Model file for the job. Use its own axes, mm. Face numbers are marked on the shaded views. A direction names the side the tool comes from. Coordinates: 2 decimals unless noted, no trailing zeros. Order: outer loops, then holes, each group sorted by start corner. A loop starts at its lowest first (then second) coordinate and runs counter-clockwise, first axis right, second up. Notation, with made-up numbers: (86.25, 77.25) -> (135.25, 77.25) arc R21 ccw to (135.25, 112.25) -> close; hole circle Ø5 at (-9.5, 54). An arc over 180 degrees is marked (long way). Return JSON: item names as keys, results as strings. Group by question number.
1) Which spindle directions (+Z, -Z, +X, -X, +Y, -Y) get a long thin tool onto all of the face, cutting with end or side? Do the marked faces 1, 2 and 3. Say none if no direction does.
2) Cut at A-A (z = 10.5). Write the cut outline in (x, y), and give its area (3 significant figures).
3) Probe line 1 (Z direction, x = 27.75, y = -19.5); line 2 (Y direction, x = 18, z = 18.5); line 3 (Y direction, x = 23.25, z = 20). List the from-to ranges inside material, lowest first.
4) Cut at B-B (z = 22.5). State how many separate pieces and enclosed holes the cut face has, and give its area (3 significant figures).
5) Flat gauge pins, fed straight in: pin 1 (1.8 mm diameter, centred on x = 11.5, z = 18.5, fed in from +Y); pin 2 (4 mm diameter, centred on x = 23, z = 0.5, fed in from -Y); pin 3 (6.5 mm diameter, centred on y = -13, z = 16.5, fed in from +X). Where does each tip first touch, or does it go through?
6) Pull direction X, two halves, no side cores. Call the marked faces 4, 5, 6 and 7: +X half, -X half, draft (parallel to the pull), parting line (faces both ways), or undercut.
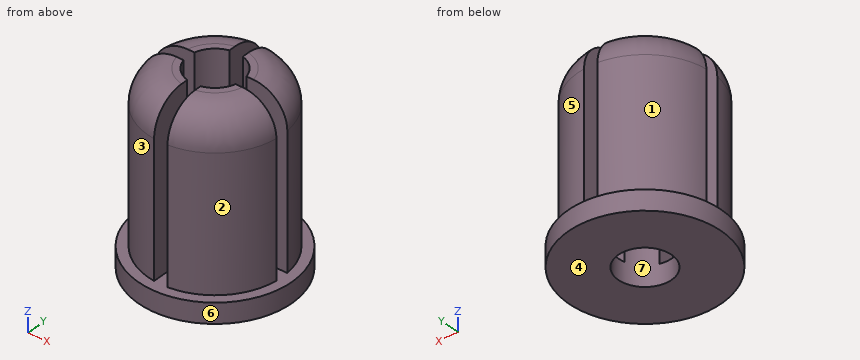
from build123d import *

# Parameters (mm, degrees)
F0_R      = 10
F0_R_2    = 4
F1_DEPTH  = 25
F2_R      = 11.5
F2_R_2    = 4
F3_DEPTH  = 3
F4_W      = 15.4053421468
F4_H      = 2
F4_W_2    = 2
F4_H_2    = 14.8476130934
F4_H_3    = 18.3621469838
F5_DEPTH  = 25
F6_R      = 5
F7_W      = 54.985769093
F7_H      = 45.2365130186
F8_DEPTH  = 25
F11_COUNT = 4
F11_ANGLE = 270


with BuildPart() as f1:
    # F0 (on Top) → F1 (new body)
    with BuildSketch(Plane.XY):
        Circle(F0_R)
        Circle(F0_R_2, mode=Mode.SUBTRACT)
    extrude(amount=F1_DEPTH)

    # F2 (on Top) → F3 (join)
    with BuildSketch(Plane.XY):
        Circle(F2_R)
        Circle(F2_R_2, mode=Mode.SUBTRACT)
    extrude(amount=-F3_DEPTH)

    # F4 (on Top) → F5 (cut)
    with BuildSketch(Plane.XY):
        with Locations((-8.7026710734, 0)):
            Rectangle(F4_W, F4_H)
        with Locations((0, 8.4238065467)):
            Rectangle(F4_W_2, F4_H_2)
        Rectangle(F4_W_2, F4_H)
        Polygon((17.6404397935, 1), (1, 1), (1, -1), (18.0223640054, -1), align=None)
        with Locations((0, -10.1810734919)):
            Rectangle(F4_W_2, F4_H_3)
    extrude(amount=F5_DEPTH, mode=Mode.SUBTRACT)

    # F6
    f6_edges = [f1.edges().sort_by_distance(p)[0] for p in [
        (7.071068, -7.071068, 25),
        (7.071068, 7.071068, 25),
        (-7.071068, 7.071068, 25),
        (-7.071068, -7.071068, 25),
    ]]
    fillet(f6_edges, radius=F6_R)


with BuildPart() as f8:
    # F7 (on Top) → F8 (new body)
    with BuildSketch(Plane.XY):
        with Locations((-82.9663015902, -56.8597912788)):
            Rectangle(F7_W, F7_H)
    extrude(amount=F8_DEPTH)


with BuildPart() as f11_1:
    # F11: instance of F1
    add(f1.part.rotate(Axis((0, -20.0353357941, 8.0697890371), (0, 0, -1)), 1 * F11_ANGLE / (F11_COUNT - 1)))


with BuildPart() as f11_2:
    # F11: instance of F1
    add(f1.part.rotate(Axis((0, -20.0353357941, 8.0697890371), (0, 0, -1)), 2 * F11_ANGLE / (F11_COUNT - 1)))


with BuildPart() as f11_3:
    # F11: instance of F1
    add(f1.part.rotate(Axis((0, -20.0353357941, 8.0697890371), (0, 0, -1)), 3 * F11_ANGLE / (F11_COUNT - 1)))


solid = f11_1.part
Answers below:
{
 "1": {"face 1": "+Z, -X, +Y", "face 2": "+Z, +X, -Y", "face 3": "+Z, -X, -Y"},
 "2": {"outline": "(10.09, -21.04) arc R10 ccw to (19.04, -29.99) -> (19.04, -23.91) arc R4 cw to (16.16, -21.04) -> close; (10.09, -19.04) -> (16.16, -19.04) arc R4 cw to (19.04, -16.16) -> (19.04, -10.09) arc R10 ccw to start; (21.04, -29.99) arc R10 ccw to (29.99, -21.04) -> (23.91, -21.04) arc R4 cw to (21.04, -23.91) -> close; (21.04, -16.16) arc R4 cw to (23.91, -19.04) -> (29.99, -19.04) arc R10 ccw to (21.04, -10.09) -> close", "area": "216 mm^2"},
 "3": {"line 1": "z = -3 to 0", "line 2": "y = -29.83 to -23.48, -16.59 to -10.24", "line 3": "y = -29.5 to -22.42, -17.66 to -10.57"},
 "4": {"separate pieces": "4", "enclosed holes": "0", "area": "180 mm^2"},
 "5": {"pin 1": "stops at y = -13.58", "pin 2": "stops at y = -31.49", "pin 3": "stops at x = 29.29"},
 "6": {"face 4": "draft", "face 5": "+X half", "face 6": "parting line", "face 7": "undercut"}
}
